Source: CAD feature listing. Evaluate the final solid. Frame: model axes, mm. Coordinates: 2 decimals unless noted, no trailing zeros. Write each loop counter-clockwise with the first axis right and the second up, starting at its lowest first coordinate (ties: lowest second). Pieces come first, ordered by that corner, then holes. Notation, with made-up numbers: M 56,67 L 66,67 A24 ccw 66,92 Z; hole C 26.25,-33 d7. An arc over 180 degrees is marked long. Write item = value, one per line. Start each with the question number.
1. Section query A-A (x = 50). Output: boundary loops of the cut face in (y, z), then the cut area to 3 significant figures.
2. Section query B-B (y = 4.25). Output: boundary loops of the cut face in (x, z), then the cut area to 3 significant figures.
3. Pin query (flat end, axial travel): pin 1 Ø5 at (y, z) = (5.5, -285) entering from +X; pin 2 Ø5 at (y, z) = (5.5, 3.5) entering from -X; pin 3 Ø1.5 at (x, y) = (73, 4) entering from -Z. Return the tip coordinate at first contact, or that it passes through.
4. Line query: line 1 along X through (y, z) = (7, -345); line 2 along Z through (x, y) = (50.5, 4); line 3 along Z through (x, y) = (56, 2.5). Output: solid intervals per line, ascending.
5. Section query C-C (x = 10). Output: boundary loops of the cut face in (y, z).
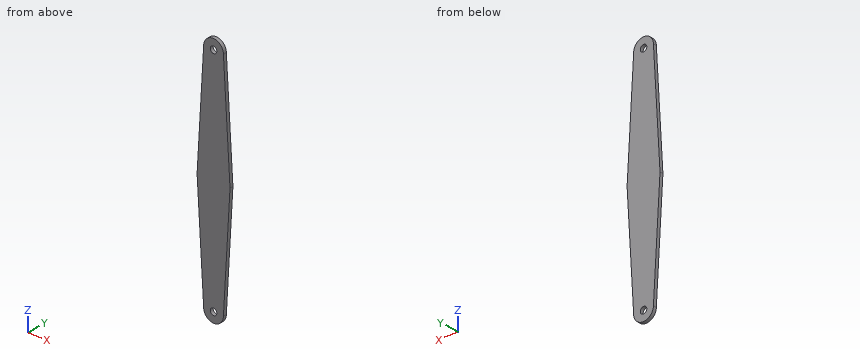
```python
from build123d import *

# Parameters (mm, degrees)
BOSS_EXTRUDE1_DEPTH = 10
SKETCH2_R           = 10
CUT_EXTRUDE1_DEPTH  = 10


with BuildPart() as part:
    # Sketch1 → Boss-Extrude1 (new body)
    with BuildSketch(Plane(origin=(0, 0, 0), x_dir=(1, 0, 0), z_dir=(0, 1, 0))):
        with BuildLine():
            Line((20, 345), (0, 0))
            Line((0, 0), (20, -345))
            ThreePointArc((20, -345), (50, -375), (80, -345))
            Line((80, -345), (100, 0))
            Line((100, 0), (80, 345))
            ThreePointArc((80, 345), (50, 375), (20, 345))
        make_face()
    extrude(amount=BOSS_EXTRUDE1_DEPTH)

    # Sketch2 → Cut-Extrude1 (cut)
    with BuildSketch(Plane(origin=(0, 10, 0), x_dir=(1, 0, 0), z_dir=(0, 1, 0))):
        with Locations(Location((50, -345, 0), (0, 0, 270))):
            Circle(SKETCH2_R)
        with Locations(Location((50, 345, 0), (0, 0, 90))):
            Circle(SKETCH2_R)
    extrude(amount=-CUT_EXTRUDE1_DEPTH, mode=Mode.SUBTRACT)


solid = part.part
```
Results are:
q1.outline = M 0,-375 L 10,-375 L 10,-355 L 0,-355 Z; M 0,-335 L 10,-335 L 10,335 L 0,335 Z; M 0,355 L 10,355 L 10,375 L 0,375 Z
q1.area = 7,100 mm^2
q2.outline = M 0,0 L 20,-345 A30 ccw 80,-345 L 100,0 L 80,345 A30 ccw 20,345 Z; hole C 50,-345 d20; hole C 50,345 d20
q2.area = 57,400 mm^2
q3.pin_1 = 83.62
q3.pin_2 = 0.06
q3.pin_3 = -365.12
q4.line_1 = 20 to 40, 60 to 80
q4.line_2 = -375 to -354.99, -335.01 to 335.01, 354.99 to 375
q4.line_3 = -374.39 to -353, -337 to 337, 353 to 374.39
q5.outline = M 0,-172.5 L 10,-172.5 L 10,172.5 L 0,172.5 Z
